For this review, use the dimensioned drawing (mm, ordinates from the lowest corner) and the shaded views. Give positions to 0.01 mm unless a question says otherwise; leave off trailing zeros. Order: outer loops, then holes, each group sorted by start corner. A loop starts at its lowest first (then second) coordinate and runs counter-clockwise, first axis right, second up. Notation, with made-up numbers: M 62,48 L 117,48 A10 ccw 117,56 Z; hole C 11,64.25 d1. An arc over 180 degrees is marked long. Use CSV: the item, a comma, the result in double quotes. Start each with the question number.
(1) Consider section B-B (z = 222). Write out the cut boundary in (x, y).
(2) Draft analysis for pull direction Z (two halves, no side actions). For the marked faces 1, 2 and 3, state which applies: pulls with the +Z half, pulls with the -Z half, needs draft (parallel to the pull), parting line crosses it, or undercut.
(3) Clearance check with flat-ended pins moving along their axes: P1, Ø4, axis at y = 11, z = 195, coming from the -X side; P2, Ø8, axis at y = 3, z = 78, coming from the +X side; P3, Ø3.5, axis at x = 33.87, z = 61.53, coming from the -Y side; P4, Ø12, axis at x = 189.5, y = 17, coming from the -Z side. State where each tip first meets the part, or that it passes through.
(4) Consider section C-C (y = 7.75). Give the number of separate pieces and of enclosed holes in the cut face, and give its area (3 significant figures).
(5) Wall thickness on L1, parallel to X at y = 7, z = 64 (1 decimal); L2, parallel to X at y = 6.75, z = 80; L3, parallel to Z at x = 42, y = 9.25 (1 decimal): over which ranges is each line inside the solid? List them lowest first. Write a range as from..to.
(6) Consider section A-A (x = 135). Write out the cut boundary in (y, z), and give its area (3 significant figures).
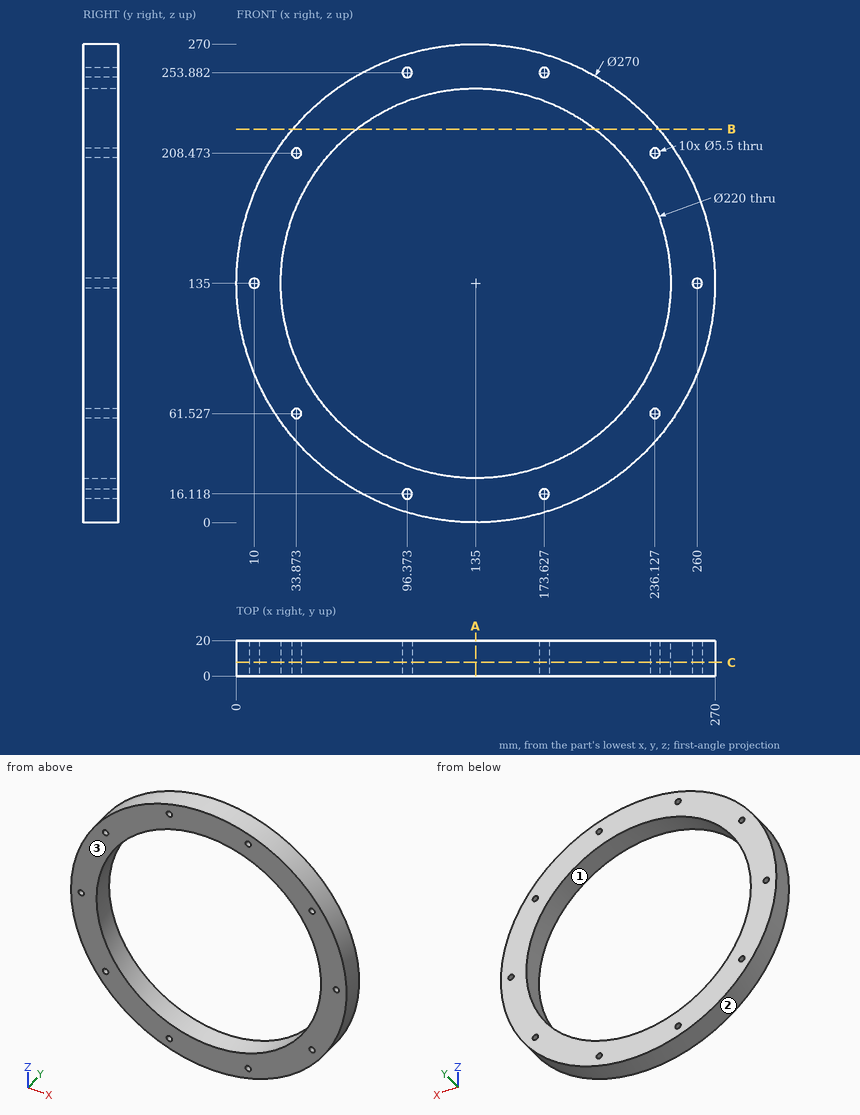
Check result:
1,outline,"M 31.77,0 L 67.69,0 L 67.69,20 L 31.77,20 Z; M 202.31,0 L 238.23,0 L 238.23,20 L 202.31,20 Z"
2,face 1,"undercut"
2,face 2,"parting line crosses it"
2,face 3,"needs draft"
3,P1,"stops at x = 13.09"
3,P2,"stops at x = 259.16"
3,P3,"passes through"
3,P4,"stops at z = 9.01"
4,separate pieces,"1"
4,enclosed holes,"11"
4,area,"19,000 mm^2"
5,L1,"x = 20.2..32.7, 35.1..51, 219..234.9, 237.3..249.8"
5,L2,"x = 11.71..39.74, 230.26..258.29"
5,L3,"z = 37.1..76.3, 193.7..232.9"
6,outline,"M 0,0 L 20,0 L 20,25 L 0,25 Z; M 0,245 L 20,245 L 20,270 L 0,270 Z"
6,area,"1,000 mm^2"
